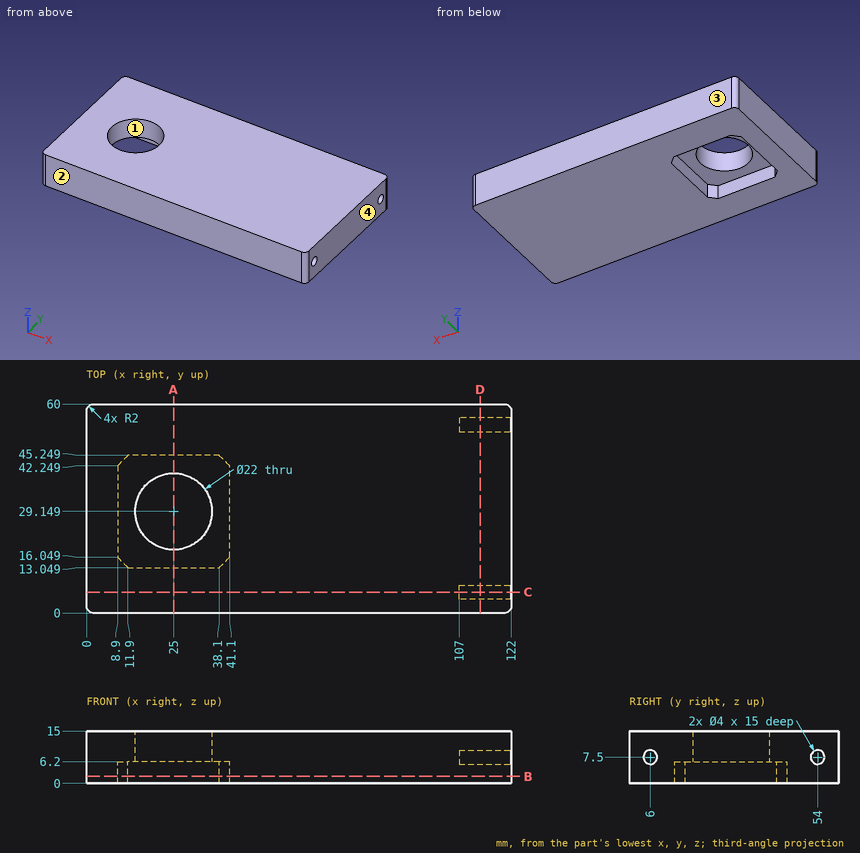
Part print with two shaded views. Sizes in mm from the minimum x, y, z corner. Round coordinates to 2 decimals unless told otherwise and drop trailing zeros. Order: outer loops, then holes, each group sorted by start corner. A loop starts at its lowest first (then second) coordinate and runs counter-clockwise, first axis right, second up. Notation, with made-up numbers: M 53,71 L 77,71 A22 cw 77,101 Z; hole C 75,42.5 d6. An arc over 180 degrees is marked long. Use CSV: the item, a comma, the result in double quotes.
Item 1: Saw through at A-A (x = 25). List the corners of the cut face in (y, z).
Worked answers:
outline,"M 0,0 L 13.05,0 L 13.05,6.2 L 18.15,6.2 L 18.15,15 L 0,15 Z; M 40.15,6.2 L 45.25,6.2 L 45.25,0 L 60,0 L 60,15 L 40.15,15 Z"
Item 2: Probe probe 1 along Y at (x, z) = (25, 11); probe 2 along Z at (x, y) = (113.5, 54); probe 3 along Y at (x, z) = (15, 2.75). List the from-to ranges inside material, lowest first.
Worked answers:
probe 1,"0 to 18.15, 40.15 to 60"
probe 2,"0 to 5.5, 9.5 to 15"
probe 3,"0 to 13.05, 45.25 to 60"
Item 3: Saw through at B-B (z = 2). List the corners of the cut face in (x, y), plus the area to 3 significant figures.
Worked answers:
outline,"M 0,2 A2 ccw 2,0 L 120,0 A2 ccw 122,2 L 122,58 A2 ccw 120,60 L 2,60 A2 ccw 0,58 Z; hole M 8.9,16.05 L 11.9,13.05 L 38.1,13.05 L 41.1,16.05 L 41.1,42.25 L 38.1,45.25 L 11.9,45.25 L 8.9,42.25 Z"
area,"6,300 mm²"
Item 4: Pull direction Y, two halves, no side cores. Call the marked faces 1, 2, 3 and 4: released by +Y, released by -Y, zero draft, split by the parting line, or undercut.
Worked answers:
face 1,"undercut"
face 2,"released by -Y"
face 3,"released by +Y"
face 4,"zero draft"
Item 5: Pin check, flat tips, straight feed: pin 1 (3.5 mm diameter, centred on y = 54, z = 7.5, fed in from +X); pin 2 (6 mm diameter, centred on x = 32, y = 17, fed in from -Z). Stop position of each tip, or through.
Worked answers:
pin 1,"x = 107"
pin 2,"z = 6.2"
Item 6: Saw through at C-C (y = 6). List the corners of the cut face in (x, z).
Worked answers:
outline,"M 0,0 L 122,0 L 122,5.5 L 107,5.5 L 107,9.5 L 122,9.5 L 122,15 L 0,15 Z"
Item 7: Saw through at D-D (x = 113). List the corners of the cut face in (y, z).
Worked answers:
outline,"M 0,0 L 60,0 L 60,15 L 0,15 Z; hole C 6,7.5 d4; hole C 54,7.5 d4"
